Check sheet for the modelled part. Datum: model origin and axes. Units: mm. Round coordinates to 2 decimals unless told otherwise and drop trailing zeros. Write each loop counter-clockwise with the first axis right and the second up, starting at its lowest first coordinate (ties: lowest second). Pieces come first, ordered by that corner, then holes.
Item 1: Release check for a two-part mould opening along X. For faces 1 (the flat face through (119, 0, 39)), 2 (the flat face through (23, 12.7, -48)), 3 (the flat face through (432.222, 13, 30)) record: +X half, -X half, draft (parallel to the pull), parting line (faces both ways), or undercut.
Item 2: Cross-section at B-B on y = 5.25. Enter the section's corners in (x, z), plus the area to 3 significant figures.
Item 3: Go/stop test with flat-tipped pins: pin 1 Ø14 at (x, y) = (21, 9) entering from -Z; pin 2 Ø3 at (x, y) = (-372, 9) entering from -Z; pin 3 Ø7.5 at (x, z) = (418.5, -139) entering from -Y. Record where each tip stops, or that it passes through.
Item 4: Material ranges on line 1 (X direction, y = 5, z = 68), recorded low to high.
Item 5: Cross-section at A-A on z = -91.5. Enter the section's corners in (x, y), plus the area to 3 significant figures.
Autodesk Inventor part; units mm, degrees
ref_plane "YZ Plane" through (0, 0, 0) normal (1, 0, 0) x (0, 1, 0)
ref_plane "XZ Plane" through (0, 0, 0) normal (0, 1, 0) x (-1, 0, 0)
ref_plane "XY Plane" through (0, 0, 0) normal (0, 0, 1) x (1, 0, 0)
sketch "Sketch1" plane through (0, 0, 0) normal (0, 1, 0) x (-1, 0, 0)
  line L0 (386.9283, -286.643) -> (-432.2217, -286.643)
  line L1 (-432.2217, -286.643) -> (-432.2217, 354.707)
  line L2 (-432.2217, 354.707) -> (386.9283, 354.707)
  line L3 (386.9283, 354.707) -> (386.9283, -286.643)
  point P0 (0, 0)
  dimension "d0" = 641.35
  dimension "d1" = 819.15
extrude "Board" add sketch "Sketch1" along normal blind 25.4
sketch "Sketch2" plane through (0, 0, 0) normal (0, -1, 0) x (1, 0, 0)
  line L0 (422.6967, -286.643) -> (413.1717, -286.643)
  line L1 (413.1717, -286.643) -> (413.1717, 183.257)
  line L2 (413.1717, 183.257) -> (422.6967, 183.257)
  line L3 (422.6967, 183.257) -> (422.6967, -286.643)
  line L4 (-367.8783, -286.643) -> (-377.4033, -286.643)
  line L5 (-377.4033, -286.643) -> (-377.4033, 183.257)
  line L6 (-377.4033, 183.257) -> (-367.8783, 183.257)
  line L7 (-367.8783, 183.257) -> (-367.8783, -286.643)
  line L8 (-386.9283, -286.643) -> (432.2217, -286.643)
  line L9 (432.2217, -286.643) -> (432.2217, 354.707)
  line L10 (-386.9283, -286.643) -> (-386.9283, 354.707)
  line L11 (13.1217, -286.643) -> (32.1717, -286.643)
  line L12 (32.1717, -286.643) -> (32.1717, 183.257)
  line L13 (32.1717, 183.257) -> (13.1217, 183.257)
  line L14 (13.1217, 183.257) -> (13.1217, -286.643)
  point P0 (0, 0)
  dimension "d4" = 469.9
  dimension "d5" = 9.525
  dimension "d6" = 9.525
  dimension "d7" = 9.525
  dimension "d10" = 19.05
  dimension "d11" = 819.15
  dimension "d12" = 400.05
  dimension "d14" = 400.05
extrude "Vertical Wall Stop Dado Notches" cut sketch "Sketch2" against normal blind 12.7
equation "\"d7\" = d6"
equation "\"d12\" = 0.5 * d11 - 0.5 * d10"
properties part number "Top"
Response values:
1. face 1: draft
1. face 2: undercut
1. face 3: +X half
2. outline: (-386.93, -286.64) - (-377.4, -286.64) - (-377.4, 183.26) - (-367.88, 183.26) - (-367.88, -286.64) - (13.12, -286.64) - (13.12, 183.26) - (32.17, 183.26) - (32.17, -286.64) - (413.17, -286.64) - (413.17, 183.26) - (422.7, 183.26) - (422.7, -286.64) - (432.22, -286.64) - (432.22, 354.71) - (-386.93, 354.71) - close
2. area: 507,000 mm2
3. pin 1: stops at z = -286.64
3. pin 2: stops at z = 183.26
3. pin 3: stops at y = 12.7
4. line 1: x = -386.93 to -377.4, -367.88 to 13.12, 32.17 to 413.17, 422.7 to 432.22
5. outline: (-386.93, 0) - (-377.4, 0) - (-377.4, 12.7) - (-367.88, 12.7) - (-367.88, 0) - (13.12, 0) - (13.12, 12.7) - (32.17, 12.7) - (32.17, 0) - (413.17, 0) - (413.17, 12.7) - (422.7, 12.7) - (422.7, 0) - (432.22, 0) - (432.22, 25.4) - (-386.93, 25.4) - close
5. area: 20,300 mm2
